Can you work these out from the model? Positions are in its coordinate system, mm. Coordinates: 2 decimals unless noted, no trailing zeros. Order: outer loops, then holes, each group sorted by start corner. A loop starts at its lowest first (then second) coordinate and runs counter-clockwise, first axis right, second up.
```python
from build123d import *

# Parameters (mm, degrees)
F1_DEPTH = 65
F2_R     = 1.75
F3_DEPTH = 65


with BuildPart() as f1:
    # F0 (on Right) → F1 (new body)
    with BuildSketch(Plane.YZ):
        with BuildLine():
            Line((37.5, -25), (37.5, 25))
            Line((37.5, 25), (-12.5, 25))
            ThreePointArc((-12.5, 25), (-37.5, 0), (-12.5, -25))
            Line((-12.5, -25), (37.5, -25))
        make_face()
    extrude(amount=F1_DEPTH)

    # F2 (on face) → F3 (cut)
    with BuildSketch(Plane.YZ.offset(65)):
        with Locations((-12.5, 0)):
            Circle(F2_R)
        with Locations((-12.5, 17.5)):
            Circle(F2_R)
        with Locations((-30, 0)):
            Circle(F2_R)
    extrude(amount=-F3_DEPTH, mode=Mode.SUBTRACT)


solid = f1.part
```
1. Imagine slicing it at A-A on z = 0. Please give me the cut outline in (x, y).
Completed:
outline: (0, -37.5) - (65, -37.5) - (65, -31.75) - (0, -31.75) - close; (0, -28.25) - (65, -28.25) - (65, -14.25) - (0, -14.25) - close; (0, -10.75) - (65, -10.75) - (65, 37.5) - (0, 37.5) - close
2. Please list where these lines run through material, in increasing order: probe 1 along Z at (x, y) = (45.5, -12.5); probe 2 along Y at (x, z) = (29.5, 0.5) (3 decimals); probe 3 along Z at (x, y) = (44, -30).
Completed:
probe 1: z = -25 to -1.75, 1.75 to 15.75, 19.25 to 25
probe 2: y = -37.495 to -31.677, -28.323 to -14.177, -10.823 to 37.5
probe 3: z = -17.85 to -1.75, 1.75 to 17.85
3. Imagine slicing it at B-B on x = 47. Please give me the cut outline in (y, z), then the cut area to 3 significant figures.
Completed:
outline: (-12.5, -25) - (37.5, -25) - (37.5, 25) - (-12.5, 25) arc R25 ccw to start; hole circle Ø3.5 at (-30, 0); hole circle Ø3.5 at (-12.5, 0); hole circle Ø3.5 at (-12.5, 17.5)
area: 3,450 mm2
4. I'm going to push flat-ended pins straight in: pin 1 (8 mm diameter, centred on x = 33, z = -13.5, fed in from -Y); pin 2 (12 mm diameter, centred on x = 14, z = 15, fed in from -Y); pin 3 (6 mm diameter, centred on x = 54.5, z = -9.5, fed in from -Y). Where does each tip first touch, or does it pass through?
Completed:
pin 1: stops at y = -35.62
pin 2: stops at y = -35.82
pin 3: stops at y = -36.64
5. Imagine slicing it at C-C on y = -30. Please give me the cut outline in (x, z), then the cut area to 3 significant figures.
Completed:
outline: (0, -17.85) - (65, -17.85) - (65, -1.75) - (0, -1.75) - close; (0, 1.75) - (65, 1.75) - (65, 17.85) - (0, 17.85) - close
area: 2,090 mm2
6. Imagine slicing it at D-D on z = 14.5. Please give me the cut outline in (x, y), then the cut area to 3 significant figures.
Completed:
outline: (0, -32.87) - (65, -32.87) - (65, 37.5) - (0, 37.5) - close
area: 4,570 mm2
7. Thinking about a two-plate mould opening in Z: for faces 1 (the flat face through (32, 12, -25)), 2 (the cylindrical face through (32.955, -10.831, 0.526)), 3 (the flat face through (65, -1, 0)), 4 (the cylindrical face through (32.045, -37.494, 0.55)), which applies, pulls with the +Z half, pulls with the -Z half, needs draft (parallel to the pull), parting line crosses it, or undercut?
Completed:
face 1: pulls with the -Z half
face 2: undercut
face 3: needs draft
face 4: parting line crosses it
